```python
from build123d import *

# Parameters (mm, degrees)
BOSS_EXTRUDE1_DEPTH            = 15
SKETCH3_R                      = 2.1
CUT_EXTRUDE2_DEPTH             = 131.149913561
SKETCH2_W                      = 125
SKETCH2_H                      = 33
BOSS_EXTRUDE4_DEPTH            = 4
SKETCH8_W                      = 7
SKETCH8_H                      = 19
BOSS_EXTRUDE5_DEPTH            = 15
CUT_EXTRUDE4_REACH             = 125.992
SKETCH6_R                      = 3.575
CUT_EXTRUDE4_DIRECTION_2_DEPTH = 124.991935222


with BuildPart() as part:
    # Sketch1 → Boss-Extrude1 (new body)
    with BuildSketch(Plane(origin=(0, 0, 0), x_dir=(1, 0, 0), z_dir=(0, 1, 0))):
        Polygon((125, 26), (125, 33), (0, 33), (0, 0), (125, 0), (125, 7), (7, 7), (7, 26), align=None)
    extrude(amount=BOSS_EXTRUDE1_DEPTH)

    # Sketch3 → Cut-Extrude2 (cut, through all)
    with BuildSketch(Plane.XY):
        with Locations((117, 8)):
            Circle(SKETCH3_R)
        with BuildLine():
            Line((82, 5.9), (32, 5.9))
            ThreePointArc((32, 5.9), (29.9, 8), (32, 10.1))
            Line((32, 10.1), (82, 10.1))
            ThreePointArc((82, 10.1), (84.1, 8), (82, 5.9))
        make_face()
    extrude(amount=-CUT_EXTRUDE2_DEPTH, mode=Mode.SUBTRACT)

    # Sketch2 → Boss-Extrude4 (add)
    with BuildSketch(Plane(origin=(0, 15, 0), x_dir=(1, 0, 0), z_dir=(0, 1, 0))):
        with Locations((62.5, 16.5)):
            Rectangle(SKETCH2_W, SKETCH2_H)
    extrude(amount=BOSS_EXTRUDE4_DEPTH)

    # Sketch8 → Boss-Extrude5 (add)
    with BuildSketch(Plane.XZ.offset(-15)):
        with Locations((93.5, -16.5)):
            Rectangle(SKETCH8_W, SKETCH8_H)
    extrude(amount=BOSS_EXTRUDE5_DEPTH)

    # Cut-Extrude4: up to this face of the body (flat: up to its plane)
    cut_extrude4_end = Plane(part.part.faces().sort_by_distance((97, 7.5, -16.5))[0])
    # Sketch6 → Cut-Extrude4 (cut, up to the picked face)
    with BuildSketch(Plane(origin=(7, 0, 0), x_dir=(0, 0, -1), z_dir=(1, 0, 0)), mode=Mode.PRIVATE) as cut_extrude4_sk1:
        with Locations(Location((16.5, 8, 0), (0, 0, 180))):
            Circle(SKETCH6_R)
    cut_extrude4_tool1 = split(extrude(cut_extrude4_sk1.sketch, amount=CUT_EXTRUDE4_REACH, mode=Mode.PRIVATE), bisect_by=cut_extrude4_end, keep=Keep.BOTH, mode=Mode.PRIVATE)
    add(cut_extrude4_tool1.solids().sort_by(Axis((7, 8, -16.5), (1, 0, 0)))[0], mode=Mode.SUBTRACT)

    # Sketch6 → Cut-Extrude4 direction 2 (cut)
    with BuildSketch(Plane(origin=(7, 0, 0), x_dir=(0, 0, -1), z_dir=(1, 0, 0))):
        with Locations(Location((16.5, 8, 0), (0, 0, 180))):
            Circle(SKETCH6_R)
    extrude(amount=-CUT_EXTRUDE4_DIRECTION_2_DEPTH, mode=Mode.SUBTRACT)


solid = part.part
```
Input: part model. Units: mm. Frame: model coordinates. A direction names the side the tool comes from. Round coordinates to 2 decimals unless told otherwise and drop trailing zeros. Order: outer loops, then holes, each group sorted by start corner. A loop starts at its lowest first (then second) coordinate and runs counter-clockwise, first axis right, second up. Notation, with made-up numbers: (-32.5, -14) - (-12.5, -14) arc R18 ccw to (-12.5, -3) - close; hole circle Ø10 at (38.25, -8). An arc over 180 degrees is marked (long way). One line per question, with ' | ' between items. Start each with the question number.
1) Cut plane B-B, the plane x = 117. Return the cut outline in (y, z), then the cut area to 3 significant figures.
2) Cut plane C-C, the plane z = -21.5. Return the cut outline in (x, y), then the cut area to 3 significant figures.
3) Pull-direction query (Y, two-part tool) for faces 4 (the cylindrical face through (84.1, 8, -3.5)), 5 (the flat face through (48, 15, -17)), 6 (the flat face through (97, 4, -17)), 7 (the cylindrical face through (29.9, 8, -3.5)); classes: +Y half, -Y half, draft (parallel to the pull), parting line (faces both ways), or undercut.
4) Set-up query: faces 1 (the flat face through (57, 10.1, -29)), 2 (the flat face through (90, 4, -17)), 3 (the flat face through (111, 7, -26)). Return all of +Z, -Z, +X, -X, +Y, -Y with unobstructed straight access to the full face (end or side cutting, diameter ignored); none if empty.
5) Ray query, probe 1 along Y at (x, z) = (92.5, -16.5) (3 decimals); probe 2 along Z at (x, y) = (25, 14.75); probe 3 along Y at (x, z) = (117, -29). Return the intervals inside material, ascending.
6) Contact query for flat-ended pins moving along their axis: P1, Ø9.5, axis at y = 8, z = -16.5, coming from the +X side; P2, Ø1, axis at y = 8.5, z = -17.5, coming from the -X side. Output: stop coordinate, or through.
7) Cut plane A-A, the plane y = 1.5. Return the cut outline in (x, z).
8) Cut plane D-D, the plane x = 86. Return the cut outline in (y, z), then the cut area to 3 significant figures.
Worked out:
1) outline: (0, -33) - (5.9, -33) - (5.9, -26) - (0, -26) - close; (0, -7) - (5.9, -7) - (5.9, 0) - (0, 0) - close; (10.1, -33) - (19, -33) - (19, 0) - (10.1, 0) - (10.1, -7) - (15, -7) - (15, -26) - (10.1, -26) - close | area: 283 mm^2
2) outline: (0, 0) - (7, 0) - (7, 15) - (90, 15) - (90, 0) - (97, 0) - (97, 15) - (125, 15) - (125, 19) - (0, 19) - close | area: 710 mm^2
3) face 4: undercut | face 5: -Y half | face 6: draft | face 7: undercut
4) face 1: +Z, -Z | face 2: -Y | face 3: +X, -Y
5) probe 1: y = 0 to 4.425, 11.575 to 19 | probe 2: z = -33 to -26, -7 to 0 | probe 3: y = 0 to 5.9, 10.1 to 19
6) P1: stops at x = 97 | P2: passes through
7) outline: (0, -33) - (125, -33) - (125, -26) - (97, -26) - (97, -7) - (125, -7) - (125, 0) - (0, 0) - close; hole (7, -26) - (90, -26) - (90, -7) - (7, -7) - close
8) outline: (0, -33) - (19, -33) - (19, 0) - (0, 0) - (0, -7) - (15, -7) - (15, -26) - (0, -26) - close | area: 342 mm^2
